```python
from build123d import *

# Parameters (mm, degrees)
F_1_5IN_SOCKET_R    = 40.64
F_1_5IN_SOCKET_R_2  = 2.1
BOSS_EXTRUDE1_DEPTH = 12.7


with BuildPart() as part:
    # 1.5in Socket → Boss-Extrude1 (new body)
    with BuildSketch(Plane(origin=(0, 0, 0), x_dir=(1, 0, 0), z_dir=(0, 1, 0))):
        with Locations(Location((0, 0, 0), (0, 0, 270))):
            Circle(F_1_5IN_SOCKET_R)
        with Locations(Location((12.927811712, 31.210498367, 0), (0, 0, 270))):
            Circle(F_1_5IN_SOCKET_R_2, mode=Mode.SUBTRACT)
        with Locations(Location((31.210498367, -12.927811712, 0), (0, 0, 270))):
            Circle(F_1_5IN_SOCKET_R_2, mode=Mode.SUBTRACT)
        with Locations(Location((-31.210498367, 12.927811712, 0), (0, 0, 270))):
            Circle(F_1_5IN_SOCKET_R_2, mode=Mode.SUBTRACT)
        with Locations(Location((-12.927811712, -31.210498367, 0), (0, 0, 270))):
            Circle(F_1_5IN_SOCKET_R_2, mode=Mode.SUBTRACT)
        with BuildLine():
            ThreePointArc((-20.506142942, 17.544892644), (-20.564786517, 20.564786517), (-17.544892644, 20.506142942))
            ThreePointArc((-17.544892644, 20.506142942), (-10.327669131, 24.933198884), (-2.093920166, 26.906145294))
            ThreePointArc((-2.093920166, 26.906145294), (0, 29.083), (2.093920166, 26.906145294))
            ThreePointArc((2.093920166, 26.906145294), (10.327669131, 24.933198884), (17.544892644, 20.506142942))
            ThreePointArc((17.544892644, 20.506142942), (20.564786517, 20.564786517), (20.506142942, 17.544892644))
            ThreePointArc((20.506142942, 17.544892644), (24.933198884, 10.327669131), (26.906145294, 2.093920166))
            ThreePointArc((26.906145294, 2.093920166), (29.083, 0), (26.906145294, -2.093920166))
            ThreePointArc((26.906145294, -2.093920166), (24.933198884, -10.327669131), (20.506142942, -17.544892644))
            ThreePointArc((20.506142942, -17.544892644), (20.564786517, -20.564786517), (17.544892644, -20.506142942))
            ThreePointArc((17.544892644, -20.506142942), (10.327669131, -24.933198884), (2.093920166, -26.906145294))
            ThreePointArc((2.093920166, -26.906145294), (0, -29.083), (-2.093920166, -26.906145294))
            ThreePointArc((-2.093920166, -26.906145294), (-10.327669131, -24.933198884), (-17.544892644, -20.506142942))
            ThreePointArc((-17.544892644, -20.506142942), (-20.564786517, -20.564786517), (-20.506142942, -17.544892644))
            ThreePointArc((-20.506142942, -17.544892644), (-24.933198884, -10.327669131), (-26.906145294, -2.093920166))
            ThreePointArc((-26.906145294, -2.093920166), (-29.083, 0), (-26.906145294, 2.093920166))
            ThreePointArc((-26.906145294, 2.093920166), (-24.933198884, 10.327669131), (-20.506142942, 17.544892644))
        make_face(mode=Mode.SUBTRACT)
    extrude(amount=BOSS_EXTRUDE1_DEPTH)


solid = part.part
```
Design review of the part built by this model. Coordinates are the model's own, in mm. Give positions to 0.01 mm unless a question says otherwise; leave off trailing zeros. Loops run counter-clockwise (first coordinate to the right, second up) from the corner with the lowest first, then second, coordinate; pieces in that order, holes last. Notation, with made-up numbers: M 66,86 L 104,86 A11 ccw 104,93 Z; hole C 78.25,87 d3. An arc over 180 degrees is marked long. Return JSON: item names as keys, results as strings. Group by question number.
Item 1: For probe 1 along X at (y, z) = (2.75, -13); probe 2 along X at (y, z) = (2.25, -14); probe 3 along X at (y, z) = (9.5, 19.5), list the stretches that pass through material, from the lowest coordinate up.
Item 2: Mouldability with a two-part tool opening along Z and no side actions: class faces 1 (the flat face through (-8, 0, 27)), 2 (the cylindrical face through (-24.887, 6.261, 10.438)), 3 (the cylindrical face through (20.6, 6.26, 20.53)), 4 (the cylindrical face through (40.294, 6.261, -5.291)) as released by +Z, released by -Z, zero draft, split by the parting line, or undercut.
Item 3: Insertion check: pin 1 Ø4 at (y, z) = (6.5, -11.5) entering from -X; pin 2 Ø2 at (x, y) = (-9.5, 3) entering from +Z; pin 3 Ø1.5 at (y, z) = (7, -22.5) entering from +X. Each pin has a flat end and moves straight along its axis. Give the tip position at first contact, or say it passes through.
Item 4: We need section C-C (y = 7.25). Give the boundary of the cut face in (x, z) (1 decimal), and give its area (3 significant figures).
Item 5: We need section D-D (x = 14). Give the boundary of the cut face in (y, z), and give its area (3 significant figures).
Item 6: We need section B-B (z = -4.5). Give the boundary of the cut face in (x, y), and give its area (3 significant figures).
Item 7: We need section A-A (x = 0). Give the boundary of the cut face in (y, z).
Output:
{
 "1": {"probe 1": "x = -38.5 to -33.31, -29.11 to -23.65, 23.65 to 38.5", "probe 2": "x = -38.15 to -33.02, -29.4 to -23.07, 23.07 to 38.15", "probe 3": "x = -35.66 to -21.14, 21.14 to 35.66"},
 "2": {"face 1": "zero draft", "face 2": "undercut", "face 3": "undercut", "face 4": "split by the parting line"},
 "3": {"pin 1": "stops at x = -39.51", "pin 2": "stops at z = 39.74", "pin 3": "stops at x = 34.33"},
 "4": {"outline": "C 0,0 d81.3; hole C -31.2,-12.9 d4.2; hole M -26.9,-2.1 A27 ccw -20.5,-17.5 A2.1 ccw long -17.5,-20.5 A27 ccw -2.1,-26.9 A2.1 ccw long 2.1,-26.9 A27 ccw 17.5,-20.5 A2.1 ccw long 20.5,-17.5 A27 ccw 26.9,-2.1 A2.1 ccw long 26.9,2.1 A27 ccw 20.5,17.5 A2.1 ccw long 17.5,20.5 A27 ccw 2.1,26.9 A2.1 ccw long -2.1,26.9 A27 ccw -17.5,20.5 A2.1 ccw long -20.5,17.5 A27 ccw -26.9,2.1 A2.1 ccw long Z; hole C -12.9,31.2 d4.2; hole C 12.9,-31.2 d4.2; hole C 31.2,12.9 d4.2", "area": "2,790 mm^2"},
 "5": {"outline": "M 0,-38.15 L 12.7,-38.15 L 12.7,-33.02 L 0,-33.02 Z; M 0,-29.4 L 12.7,-29.4 L 12.7,-23.07 L 0,-23.07 Z; M 0,23.07 L 12.7,23.07 L 12.7,38.15 L 0,38.15 Z", "area": "337 mm^2"},
 "6": {"outline": "M -40.39,0 L -26.61,0 L -26.61,12.7 L -40.39,12.7 Z; M 26.61,0 L 40.39,0 L 40.39,12.7 L 26.61,12.7 Z", "area": "350 mm^2"},
 "7": {"outline": "M 0,-40.64 L 12.7,-40.64 L 12.7,-29.08 L 0,-29.08 Z; M 0,29.08 L 12.7,29.08 L 12.7,40.64 L 0,40.64 Z"}
}
